Autodesk Inventor part; units mm, degrees
ref_plane "YZ Plane" through (0, 0, 0) normal (1, 0, 0) x (0, 1, 0)
ref_plane "XZ Plane" through (0, 0, 0) normal (0, 1, 0) x (-1, 0, 0)
ref_plane "XY Plane" through (0, 0, 0) normal (0, 0, 1) x (1, 0, 0)
sketch "Sketch1" plane through (0, 0, 0) normal (1, 0, 0) x (0, 1, 0)
  line L0 (0, 0) -> (50.8, 0)
  line L1 (50.8, 0) -> (50.8, -82.55)
  line L2 (50.8, -82.55) -> (0, -82.55)
  line L3 (0, -82.55) -> (0, -57.15)
  line L4 (0, -57.15) -> (-10.16, -57.15)
  line L5 (-10.16, -57.15) -> (-10.16, 0)
  line L6 (-10.16, 0) -> (0, 0)
  dimension "d0" = 82.55
  dimension "d1" = 50.8
  dimension "d27" = 25.4
  dimension "d28" = 10.16
extrude "Extrusion1" add sketch "Sketch1" along normal blind 6.35
sketch "Sketch2" plane through (6.35, 0, 0) normal (1, 0, 0) x (0, 0, -1)
  circle A0 centre (55.88, 8.89) radius 2.54
  line L0 (0, 0) -> (25.4, 0)
  line L1 (0, 50.8) -> (0, 0)
  line L2 (57.15, -10.16) -> (57.15, 0)
  arc A1 (14.5266, 38.3949) -> (7.2244, -5.7138) centre (55.88, 8.89) ccw construction
  arc A2 (12.459, 39.8702) -> (4.7916, -6.444) centre (55.88, 8.89) ccw
  arc A3 (16.5943, 36.9197) -> (9.6572, -4.9836) centre (55.88, 8.89) ccw
  arc A4 (16.5943, 36.9197) -> (12.459, 39.8702) centre (14.5266, 38.3949) ccw
  arc A5 (4.7916, -6.444) -> (9.6572, -4.9836) centre (7.2244, -5.7138) ccw
  point P0 (82.55, 0)
  dimension "d4" = 8.89
  dimension "d7" = 5.08
  dimension "d43" = 1.27
  dimension "d44" = 52.214
  dimension "d46" = 2.54
  dimension "d47" = 50.8
extrude "Extrusion2" cut sketch "Sketch2" against normal through all
sketch "Sketch6" plane through (0, 0, -82.55) normal (0, -1, 0) x (1, 0, 0)
  line L0 (0, 0) -> (0, 25.4)
  line L1 (0, 0) -> (0, 25.4)
  line L2 (0, 0) -> (6.35, 0)
  line L3 (6.35, 25.4) -> (6.35, 0)
  line L4 (0, 25.4) -> (6.35, 25.4)
  point P0 (0, 82.55)
  point P1 (3.175, 12.7)
sketch "Sketch7" plane through (0, -10.16, 0) normal (0, 0, 1) x (1, 0, 0)
  line L0 (0, 0) -> (0, 60.96)
  line L1 (0, 0) -> (6.35, 0)
  line L2 (6.35, 60.96) -> (6.35, 0)
  line L3 (0, 60.96) -> (6.35, 60.96)
  point P0 (0, 10.16)
  point P1 (3.3657, 7.358)
  point P2 (3.175, 55.3802)
hole "Hole2" at (3.175, 0, -69.85) direction (0, 1, 0) diameter 1.9304 depth 7.6708 tip angle 118
hole "Hole3" at (3.3657, -2.802, 0) at (3.175, 45.2202, 0) direction (0, 0, -1) diameter 1.9304 depth 7.6708 tip angle 118
properties part number "third odomitry wheel"
Geometry: final body of the model. Coordinates: model frame, mm. A direction names the side the tool comes from. Coordinates: 2 decimals unless noted, no trailing zeros. Order: outer loops, then holes, each group sorted by start corner. A loop starts at its lowest first (then second) coordinate and runs counter-clockwise, first axis right, second up. Notation, with made-up numbers: (34.5, -11) -> (77.5, -11) arc R17 ccw to (77.5, 12) -> close; hole circle Ø5 at (-28.75, 73). An arc over 180 degrees is marked (long way). Write item = value, one per line.
(1) Cut plane C-C on x = 1. Return loops of the section in (y, z).
Solved:
outline = (-10.16, -57.15) -> (0, -57.15) -> (0, -82.55) -> (50.8, -82.55) -> (50.8, 0) -> (-10.16, 0) -> close; hole (-6.44, -4.79) arc R2.54 ccw to (-4.98, -9.66) arc R48.26 cw to (36.92, -16.59) arc R2.54 ccw to (39.87, -12.46) arc R53.34 ccw to start; hole circle Ø5.08 at (8.89, -55.88)
(2) Pull-direction query (X, two-part tool) for faces 4 (the flat face through (3, -10.16, -29)), 5 (the conical face through (3.111, 45.065, -8.15)), 6 (the flat face through (6.35, 20, -41)); classes: pulls with the +X half, pulls with the -X half, needs draft (parallel to the pull), parting line crosses it, or undercut.
Solved:
face_4 = needs draft
face_5 = undercut
face_6 = pulls with the +X half
(3) Cut plane D-D on y = 10. Return loops of the section in (x, z).
Solved:
outline = (0, -82.55) -> (6.35, -82.55) -> (6.35, -58.16) -> (0, -58.16) -> close; (0, -53.6) -> (6.35, -53.6) -> (6.35, -7.63) -> (0, -7.63) -> close; (0, -2.55) -> (6.35, -2.55) -> (6.35, 0) -> (0, 0) -> close
(4) Pin query (flat end, axial travel): pin 1 Ø1 at (x, z) = (5, -70.5) entering from -Y; pin 2 Ø1.2 at (x, y) = (3.37, -2.8) entering from -Z; pin 3 Ø1.5 at (x, y) = (3.18, 45.22) entering from +Z. Return the tip coordinate at first contact, or that it passes through.
Solved:
pin_1 = 0
pin_2 = -57.15
pin_3 = -7.8
(5) Cut plane A-A on z = -55.88. Return loops of the section in (x, y), plus the area to 3 significant figures.
Solved:
outline = (0, -10.16) -> (6.35, -10.16) -> (6.35, 6.35) -> (0, 6.35) -> close; (0, 11.43) -> (6.35, 11.43) -> (6.35, 50.8) -> (0, 50.8) -> close
area = 355 mm²
(6) Cut plane B-B on y = -1. Return loops of the section in (x, z).
Solved:
outline = (0, -57.15) -> (6.35, -57.15) -> (6.35, -8.64) -> (0, -8.64) -> close; (0, -3.46) -> (6.35, -3.46) -> (6.35, 0) -> (0, 0) -> close
(7) Access query for faces 1 (the cylindrical face through (3.076, -3.723, -2.06)), 2 (the cylindrical face through (3.22, 17.08, -8.32)), 3 (the cylindrical face through (3.133, 3.889, -68.886)). Directions: +Z, -Z, +X, -X, +Y, -Y. A direction counts if a zero-diameter tool reaches every point of the face in a straight line with its end or side. Return the directions, or none.
Solved:
face_1 = +Z
face_2 = +X, -X
face_3 = -Y
(8) Line query: line 1 (X direction, y = 6, z = -69.85); line 2 (Z direction, x = 2.75, y = 40); line 3 (Y direction, x = 2, z = -54). Output: solid intervals per line, ascending.
Solved:
line_1 = 0 to 2.21, 4.14 to 6.35
line_2 = -82.55 to -16.5, -12.56 to 0
line_3 = -10.16 to 7.18, 10.6 to 50.8
